Read the model definition and answer for the solid it produces. Units are mm, in the model's axes. Face numbers are marked on the shaded views. A direction names the side the tool comes from. Coordinates: 2 decimals unless noted, no trailing zeros. Write each loop counter-clockwise with the first axis right and the second up, starting at its lowest first coordinate (ties: lowest second). Pieces come first, ordered by that corner, then holes. Notation, with made-up numbers: (22.5, 79.5) - (42.5, 79.5) arc R20 cw to (42.5, 114.5) - close; hole circle Ø4 at (21, 88). An arc over 180 degrees is marked (long way). Return JSON: item names as keys, results as strings.
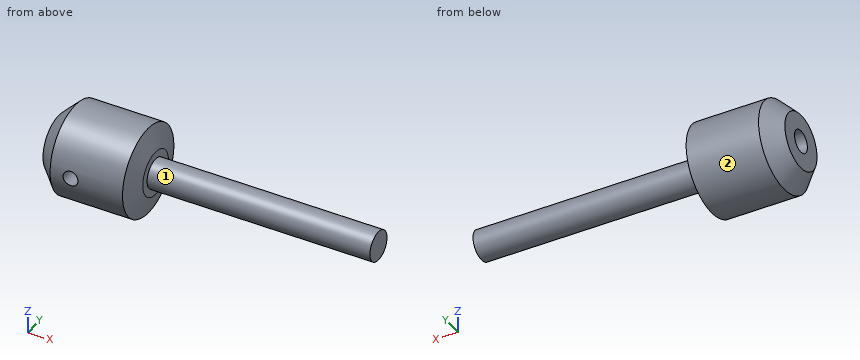
```python
from build123d import *

# Parameters (mm, degrees)
F2_R     = 1
F3_DEPTH = 10
F4_SIZE2 = 1
F4_SIZE  = 3


with BuildPart() as f1:
    # F0 (on Front) → F1 (revolve)
    with BuildSketch(Plane.XZ):
        Polygon((-33, 0), (0, 0), (0, 2), (-30, 2), (-30, 6), (-40.75, 6), (-43, 3.75), (-43, 1.5), (-33, 1.5), align=None)
    revolve(axis=Axis((-16.5, 0, 0), (-1, 0, 0)))

    # F2 (on Front) → F3 (cut)
    with BuildSketch(Plane.XZ):
        with Locations((-38, 0)):
            Circle(F2_R)
    extrude(amount=F3_DEPTH, mode=Mode.SUBTRACT)

    # F4
    f4_edges = [f1.edges().sort_by_distance(p)[0] for p in [
        (-30, 0, -6),
    ]]
    chamfer(f4_edges, length=F4_SIZE, length2=F4_SIZE2)


solid = f1.part
```
(1) A cutting plane is placed at A-A (z = 0). Determine the outline of the cut face in (x, y).
Answer:
{"outline": "(-43, -3.75) - (-40.75, -6) - (-39, -6) - (-39, -1.5) - (-43, -1.5) - close; (-43, 1.5) - (-33, 1.5) - (-33, -1.5) - (-37, -1.5) - (-37, -6) - (-31, -6) - (-30, -3) - (-30, -2) - (0, -2) - (0, 2) - (-30, 2) - (-30, 3) - (-31, 6) - (-40.75, 6) - (-43, 3.75) - close"}
(2) A cutting plane is placed at D-D (x = -15). Determine the outline of the cut face in (y, z), and give its area (3 significant figures).
Answer:
{"outline": "circle Ø4 at (0, 0)", "area": "12.6 mm²"}
(3) Which of the six approach directions +Z, -Z, +X, -X, +Y, -Y give full straight-line access (tool end or side, diameter ignored) to the marked faces 1 and 2?
Answer:
{"face 1": "+X", "face 2": "+X, -X"}
(4) A cutting plane is placed at C-C (x = -35.5). Determine the outline of the cut face in (y, z), and give its area (3 significant figures).
Answer:
{"outline": "circle Ø12 at (0, 0); hole circle Ø3 at (0, 0)", "area": "106 mm²"}
(5) Flat-ended cylindrical pins translate along their axes: P1, Ø0.9, axis at y = 0, z = -0.5, coming from the -X side; P2, Ø5, axis at x = -10.5, y = -3.5, coming from the -Z side; P3, Ø4, axis at x = -14.5, z = -3.5, coming from the -Y side. Find the tip coordinate at first contact, or state that the pin passes through.
Answer:
{"P1": "x = -33", "P2": "z = -1.73", "P3": "y = -1.32"}
(6) A cutting plane is placed at B-B (y = 0). Determine the outline of the cut face in (x, z), and give its area (3 significant figures).
Answer:
{"outline": "(-43, -3.75) - (-40.75, -6) - (-31, -6) - (-30, -3) - (-30, -2) - (0, -2) - (0, 2) - (-30, 2) - (-30, 3) - (-31, 6) - (-40.75, 6) - (-43, 3.75) - (-43, 1.5) - (-33, 1.5) - (-33, -1.5) - (-43, -1.5) - close", "area": "238 mm²"}
(7) Straight lines are drawn through the part: line 1 (X direction, y = -2.65, z = 0); line 2 (Y direction, x = -35, z = 0); line 3 (Z direction, x = -38, y = -4.45). For each, find the intervals that lie inside material, in ascending order. Write a range as from..to.
Answer:
{"line 1": "-43..-39, -37..-30", "line 2": "-6..-1.5, 1.5..6", "line 3": "-4.02..-1, 1..4.02"}
